Drawing for the job (mm, zero at the part's lowest x, y, z). A direction names the side the tool comes from. Give positions to 0.01 mm unless a question says otherwise; leave off trailing zeros. Loops run counter-clockwise (first coordinate to the right, second up) from the corner with the lowest first, then second, coordinate; pieces in that order, holes last. Notation, with made-up numbers: (-5, 1.25) - (38, 1.25) arc R25 cw to (38, 21.25) - close; hole circle Ø9 at (11.25, 80.5). An arc over 180 degrees is marked (long way). Return JSON: item names as keys, results as strings. Group by question number.
1) Slice it at B-B (y = 4.5). Count the separate pieces of the cut face and the enclosed holes in it.
2) Slice it at C-C (z = 3). List the corners of the cut face in (x, y).
3) 3-axis set-ups, long thin cutter, end or side, ignore diameter. For the marked faces 4 and 5: which of +Z, -Z, +X, -X, +Y, -Y reach the whole face in a straight line?
4) Mould opens along X. For the marked faces 1, 2 and 3 say: released by +X, released by -X, zero draft, split by the parting line, or undercut.
5) Slice it at A-A (y = 11.5). List the corners of the cut face in (x, z).
6) Drop a flat-ended pin along its axis: pin 1 (1.8 mm diameter, centred on x = 13.5, z = 1.5, fed in from -Y). Give the stop position or say it passes through.
7) Slice it at D-D (x = 3). List the corners of the cut face in (y, z).
8) Drill centre lines: probe 1 along X at (y, z) = (15.75, 0.6); probe 2 along Y at (x, z) = (13.25, 1.75); probe 3 along Y at (x, z) = (2.5, 2.05). Where is each one in solid material? Low to high. Write a range as from..to.
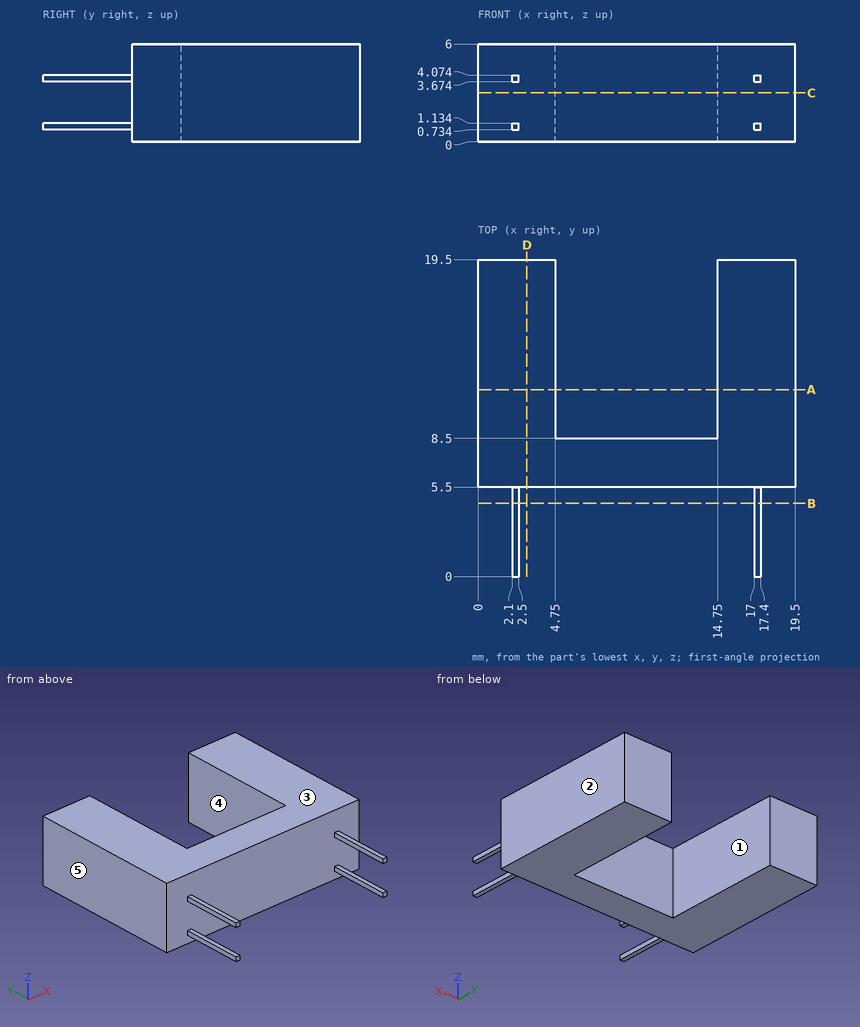
Results:
{
 "1": {"separate pieces": "4", "enclosed holes": "0"},
 "2": {"outline": "(0, 5.5) - (19.5, 5.5) - (19.5, 19.5) - (14.75, 19.5) - (14.75, 8.5) - (4.75, 8.5) - (4.75, 19.5) - (0, 19.5) - close"},
 "3": {"face 4": "+Z, -Z, +Y", "face 5": "+Z, -Z, -X, +Y, -Y"},
 "4": {"face 1": "undercut", "face 2": "released by +X", "face 3": "zero draft"},
 "5": {"outline": "(0, 0) - (4.75, 0) - (4.75, 6) - (0, 6) - close; (14.75, 0) - (19.5, 0) - (19.5, 6) - (14.75, 6) - close"},
 "6": {"pin 1": "y = 5.5"},
 "7": {"outline": "(5.5, 0) - (19.5, 0) - (19.5, 6) - (5.5, 6) - close"},
 "8": {"probe 1": "0..4.75, 14.75..19.5", "probe 2": "5.5..8.5", "probe 3": "5.5..19.5"}
}
